Design review of the part built by this model. Coordinates are the model's own, in mm. Round coordinates to 2 decimals unless told otherwise and drop trailing zeros. Write each loop counter-clockwise with the first axis right and the second up, starting at its lowest first coordinate (ties: lowest second). Pieces come first, ordered by that corner, then holes.
from build123d import *

# Parameters (mm, degrees)
SKETCH1_W           = 1500
SKETCH1_H           = 1000
SKETCH1_R           = 75
BOSS_EXTRUDE1_DEPTH = 100
CHAMFER1_SIZE       = 100


with BuildPart() as part:
    # Sketch1 → Boss-Extrude1 (new body)
    with BuildSketch(Plane.XY):
        Rectangle(SKETCH1_W, SKETCH1_H)
        with Locations((-120, 120)):
            Circle(SKETCH1_R, mode=Mode.SUBTRACT)
        with Locations((120, 120)):
            Circle(SKETCH1_R, mode=Mode.SUBTRACT)
        with Locations((120, -120)):
            Circle(SKETCH1_R, mode=Mode.SUBTRACT)
        with Locations((-120, -120)):
            Circle(SKETCH1_R, mode=Mode.SUBTRACT)
    extrude(amount=BOSS_EXTRUDE1_DEPTH)

    # Chamfer1
    # the kernel refuses this chamfer: 100 mm, written as the material it takes off along each edge
    with BuildSketch(Plane(origin=(-120, 120, 100), x_dir=(1, 0, 0), z_dir=(0, -1, 0))) as chamfer1_piece_1:
        Polygon((75, -CHAMFER1_SIZE), (75 + CHAMFER1_SIZE, 0), (75, 0), align=None)
    revolve(axis=Axis((-120, 120, 100), (0, 0, 1)), mode=Mode.SUBTRACT)
    with BuildSketch(Plane(origin=(120, 120, 100), x_dir=(1, 0, 0), z_dir=(0, -1, 0))) as chamfer1_piece_2:
        Polygon((75, -CHAMFER1_SIZE), (75 + CHAMFER1_SIZE, 0), (75, 0), align=None)
    revolve(axis=Axis((120, 120, 100), (0, 0, 1)), mode=Mode.SUBTRACT)
    with BuildSketch(Plane(origin=(120, -120, 100), x_dir=(1, 0, 0), z_dir=(0, -1, 0))) as chamfer1_piece_3:
        Polygon((75, -CHAMFER1_SIZE), (75 + CHAMFER1_SIZE, 0), (75, 0), align=None)
    revolve(axis=Axis((120, -120, 100), (0, 0, 1)), mode=Mode.SUBTRACT)
    with BuildSketch(Plane(origin=(-120, -120, 100), x_dir=(1, 0, 0), z_dir=(0, -1, 0))) as chamfer1_piece_4:
        Polygon((75, -CHAMFER1_SIZE), (75 + CHAMFER1_SIZE, 0), (75, 0), align=None)
    revolve(axis=Axis((-120, -120, 100), (0, 0, 1)), mode=Mode.SUBTRACT)


solid = part.part
1) Add section B-B on y = -120. State the section outline as (x, z) points, and give its area (3 significant figures).
2) Add section A-A on z = 73. State the section outline as (x, y) points.
3) The part is to be moulded in two halves that separate along Y. For faces 1 (the face through (-750, -7, 49)), 2 (the face through (163.682, 188.515, 6.256)), 3 (the face through (-10, -500, 49)), say which applies: pulls with the +Y half, pulls with the -Y half, needs draft (parallel to the pull), parting line crosses it, or undercut.
4) Add section C-C on x = -120. State the section outline as (y, z) points, and give its area (3 significant figures).
5) For line 1 along Y through (x, z) = (67, 49); line 2 along Y through (x, z) = (-125.5, 4.5); line 3 along X through (y, z) = (-115, 7), list the stretches that pass through material, from the lowest coordinate up.
Computed:
1. outline: (-750, 0) - (-195, 0) - (-295, 100) - (-750, 100) - close; (-45, 0) - (45, 0) - (0, 45) - close; (195, 0) - (750, 0) - (750, 100) - (295, 100) - close
1. area: 103,000 mm2
2. outline: (-750, -500) - (750, -500) - (750, 500) - (-750, 500) - close; (-33.37, 0) arc R148 cw to (0, -33.37) arc R148 cw to (33.37, 0) arc R148 cw to (0, 33.37) arc R148 cw to start; hole (-206.63, 0) arc R148 ccw (long way) to (0, -206.63) arc R148 ccw (long way) to (206.63, 0) arc R148 ccw (long way) to (0, 206.63) arc R148 ccw (long way) to start
3. face 1: needs draft
3. face 2: undercut
3. face 3: pulls with the -Y half
4. outline: (-500, 0) - (-195, 0) - (-295, 100) - (-500, 100) - close; (-45, 0) - (45, 0) - (0, 45) - close; (195, 0) - (500, 0) - (500, 100) - (295, 100) - close
4. area: 53,000 mm2
5. line 1: y = -500 to -232.1, -7.9 to 7.9, 232.1 to 500
5. line 2: y = -500 to -199.31, -40.69 to 40.69, 199.31 to 500
5. line 3: x = -750 to -201.85, -38.15 to 38.15, 201.85 to 750
